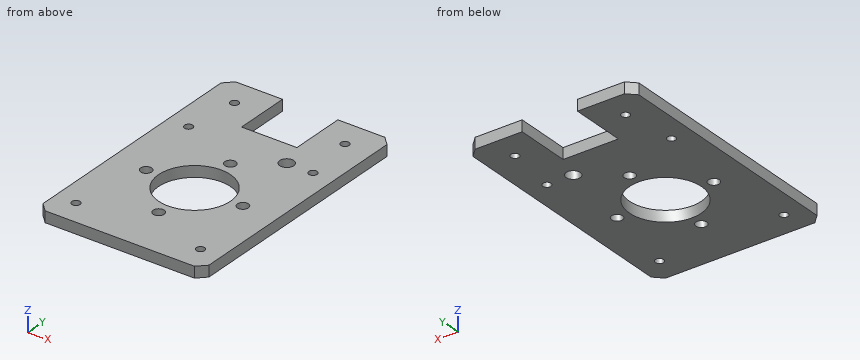
from build123d import *

# Parameters (mm, degrees)
SKETCH1_W           = 60
SKETCH1_H           = 73
BOSS_EXTRUDE1_DEPTH = 6
SKETCH2_R           = 8
CUT_EXTRUDE1_DEPTH  = 95.683683917
SKETCH3_R           = 1.5
CUT_EXTRUDE2_DEPTH  = 95.683683917
SKETCH4_R           = 21
CUT_EXTRUDE3_DEPTH  = 4
SKETCH5_W           = 20
SKETCH5_H           = 20
BOSS_EXTRUDE2_DEPTH = 6
SKETCH6_R           = 1.5
CUT_EXTRUDE4_DEPTH  = 10
CHAMFER1_SIZE       = 3
CHAMFER2_SIZE       = 3
SKETCH7_R           = 2
CUT_EXTRUDE5_DEPTH  = 111.747460467
SKETCH8_R           = 13
CUT_EXTRUDE6_DEPTH  = 111.747460467
BOSS_EXTRUDE3_START = 4
SKETCH9_R           = 21
SKETCH9_R_2         = 2
SKETCH9_R_3         = 13
BOSS_EXTRUDE3_DEPTH = 4
CUT_EXTRUDE7_DEPTH  = 2
SKETCH12_R          = 2.55
CUT_EXTRUDE8_DEPTH  = 10


with BuildPart() as part:
    # Sketch1 → Boss-Extrude1 (new body)
    with BuildSketch(Plane.XY):
        with Locations((30, 36.5)):
            Rectangle(SKETCH1_W, SKETCH1_H)
    extrude(amount=BOSS_EXTRUDE1_DEPTH)

    # Sketch2 → Cut-Extrude1 (cut, through all)
    with BuildSketch(Plane(origin=(0, 0, 0), x_dir=(-1, 0, 0), z_dir=(0, 0, -1))):
        with Locations((-30, 36.5)):
            Circle(SKETCH2_R)
    extrude(amount=-CUT_EXTRUDE1_DEPTH, mode=Mode.SUBTRACT)

    # Sketch3 → Cut-Extrude2 (cut, through all)
    with BuildSketch(Plane(origin=(0, 0, 0), x_dir=(-1, 0, 0), z_dir=(0, 0, -1))):
        with Locations((-52.5, 64)):
            Circle(SKETCH3_R)
        with Locations((-7.5, 64)):
            Circle(SKETCH3_R)
        with Locations((-52.5, 9)):
            Circle(SKETCH3_R)
        with Locations((-7.5, 9)):
            Circle(SKETCH3_R)
    extrude(amount=-CUT_EXTRUDE2_DEPTH, mode=Mode.SUBTRACT)

    # Sketch4 → Cut-Extrude3 (cut)
    with BuildSketch(Plane(origin=(0, 0, 0), x_dir=(-1, 0, 0), z_dir=(0, 0, -1))):
        with Locations((-30, 36.5)):
            Circle(SKETCH4_R)
    extrude(amount=-CUT_EXTRUDE3_DEPTH, mode=Mode.SUBTRACT)

    # Sketch5 → Boss-Extrude2 (add)
    with BuildSketch(Plane(origin=(0, 0, 0), x_dir=(-1, 0, 0), z_dir=(0, 0, -1))):
        with Locations((-50, 83)):
            Rectangle(SKETCH5_W, SKETCH5_H)
        with Locations((-10, 83)):
            Rectangle(SKETCH5_W, SKETCH5_H)
    extrude(amount=-BOSS_EXTRUDE2_DEPTH)

    # Sketch6 → Cut-Extrude4 (cut)
    with BuildSketch(Plane(origin=(0, 0, 0), x_dir=(-1, 0, 0), z_dir=(0, 0, -1))):
        with Locations((-10, 83)):
            Circle(SKETCH6_R)
        with Locations((-50, 83)):
            Circle(SKETCH6_R)
    extrude(amount=-CUT_EXTRUDE4_DEPTH, mode=Mode.SUBTRACT)

    # Chamfer1
    chamfer1_edges = [part.edges().sort_by_distance(p)[0] for p in [
        (60, 0, 3),
        (0, 0, 3),
    ]]
    chamfer(chamfer1_edges, length=CHAMFER1_SIZE)

    # Chamfer2
    chamfer2_edges = [part.edges().sort_by_distance(p)[0] for p in [
        (60, 93, 3),
        (0, 93, 3),
    ]]
    chamfer(chamfer2_edges, length=CHAMFER2_SIZE)

    # Sketch7 → Cut-Extrude5 (cut, through all)
    with BuildSketch(Plane(origin=(0, 0, 4), x_dir=(-1, 0, 0), z_dir=(0, 0, -1))):
        with Locations((-30, 54)):
            Circle(SKETCH7_R)
        with Locations((-12.5, 36.5)):
            Circle(SKETCH7_R)
        with Locations((-30, 19)):
            Circle(SKETCH7_R)
        with Locations((-47.5, 36.5)):
            Circle(SKETCH7_R)
    extrude(amount=-CUT_EXTRUDE5_DEPTH, mode=Mode.SUBTRACT)

    # Sketch8 → Cut-Extrude6 (cut, through all)
    with BuildSketch(Plane(origin=(0, 0, 4), x_dir=(-1, 0, 0), z_dir=(0, 0, -1))):
        with Locations((-30, 36.5)):
            Circle(SKETCH8_R)
    extrude(amount=-CUT_EXTRUDE6_DEPTH, mode=Mode.SUBTRACT)

    # Sketch9 → Boss-Extrude3 (add)
    with BuildSketch(Plane(origin=(0, 0, 4), x_dir=(-1, 0, 0), z_dir=(0, 0, -1)).offset(BOSS_EXTRUDE3_START)):
        with Locations((-30, 36.5)):
            Circle(SKETCH9_R)
        with Locations((-30, 54)):
            Circle(SKETCH9_R_2, mode=Mode.SUBTRACT)
        with Locations((-30, 19)):
            Circle(SKETCH9_R_2, mode=Mode.SUBTRACT)
        with Locations((-47.5, 36.5)):
            Circle(SKETCH9_R_2, mode=Mode.SUBTRACT)
        with Locations((-12.5, 36.5)):
            Circle(SKETCH9_R_2, mode=Mode.SUBTRACT)
        with Locations((-30, 36.5)):
            Circle(SKETCH9_R_3, mode=Mode.SUBTRACT)
    extrude(amount=-BOSS_EXTRUDE3_DEPTH)

    # Sketch11 → Cut-Extrude7 (cut)
    with BuildSketch(Plane.XY.offset(6)):
        Polygon((60, 3), (60, 90), (57, 93), (40, 93), (40, 73), (20, 73), (20, 93), (3, 93), (0, 90), (0, 3), (3, 0), (57, 0), align=None)
    extrude(amount=-CUT_EXTRUDE7_DEPTH, mode=Mode.SUBTRACT)

    # Sketch12 → Cut-Extrude8 (cut)
    with BuildSketch(Plane.XY.offset(4)):
        with Locations((43, 64)):
            Circle(SKETCH12_R)
    extrude(amount=-CUT_EXTRUDE8_DEPTH, mode=Mode.SUBTRACT)


solid = part.part
Geometry: final body of the model. Coordinates: model frame, mm. Give positions to 0.01 mm unless a question says otherwise; leave off trailing zeros. Order: outer loops, then holes, each group sorted by start corner. A loop starts at its lowest first (then second) coordinate and runs counter-clockwise, first axis right, second up. Notation, with made-up numbers: (62, 9.5) -> (70, 9.5) arc R36 cw to (70, 48.5) -> close; hole circle Ø1 at (68.25, 56). An arc over 180 degrees is marked (long way). Answer as a JSON object with one key per item and string values.
Q1. Section A-A (y = 9). Output: boundary loops of the cut face in (x, z), plus the area to 3 significant figures.
Entries:
{"outline": "(0, 0) -> (6, 0) -> (6, 4) -> (0, 4) -> close; (9, 0) -> (51, 0) -> (51, 4) -> (9, 4) -> close; (54, 0) -> (60, 0) -> (60, 4) -> (54, 4) -> close", "area": "216 mm^2"}
Q2. Section B-B (x = 7.5). Output: boundary loops of the cut face in (y, z), plus the area to 3 significant figures.
Entries:
{"outline": "(0, 0) -> (7.5, 0) -> (7.5, 4) -> (0, 4) -> close; (10.5, 0) -> (62.5, 0) -> (62.5, 4) -> (10.5, 4) -> close; (65.5, 0) -> (93, 0) -> (93, 4) -> (65.5, 4) -> close", "area": "348 mm^2"}
Q3. First-contact query: pin 1 (3.5 mm diameter, centred on x = 52.5, y = 64, fed in from +Z); pin 2 (2.5 mm diameter, centred on x = 7.5, y = 9, fed in from +Z); pin 3 (2 mm diameter, centred on x = 21.5, z = 2.5, fed in from +Y). Flat tips, straight axial feed; report the tip coordinate or a pass-through.
Entries:
{"pin 1": "stops at z = 4", "pin 2": "passes through", "pin 3": "stops at y = 73"}
Q4. Section C-C (z = 1.15). State how many separate pieces and enclosed holes the cut face has, plus the area to 3 significant figures.
Entries:
{"separate pieces": "1", "enclosed holes": "12", "area": "4,520 mm^2"}
Q5. Section D-D (y = 76). Output: boundary loops of the cut face in (x, z), plus the area to 3 significant figures.
Entries:
{"outline": "(0, 0) -> (20, 0) -> (20, 4) -> (0, 4) -> close; (40, 0) -> (60, 0) -> (60, 4) -> (40, 4) -> close", "area": "160 mm^2"}
Q6. Material intervals for probe 1 along Y at (x, z) = (30, 1.7); probe 2 along X at (y, z) = (87, 3.15); probe 3 along X at (y, z) = (55.5, 2.25), sorted ascending.
Entries:
{"probe 1": "y = 0 to 17, 21 to 23.5, 49.5 to 52, 56 to 73", "probe 2": "x = 0 to 20, 40 to 60", "probe 3": "x = 0 to 28.68, 31.32 to 60"}
